```python
from build123d import *

# Parameters (mm, degrees)
F1_DEPTH = 15
F2_W     = 12
F2_H     = 14
F3_DEPTH = 7.5
F4_W     = 11
F4_H     = 14
F5_DEPTH = 17
F6_W     = 11
F6_H     = 1.5
F7_DEPTH = 5.2


with BuildPart() as f1:
    # F0 (on Right) → F1 (new body)
    with BuildSketch(Plane.YZ):
        Polygon((-17, 0), (0, 0), (0, 7.5), (-4, 7.5), (-4, 17), (-8.5, 17), (-8.5, 14), (-6, 14), (-6, 10), (-11.8, 10), (-11.8, 17), (-17, 11.8), align=None)
    extrude(amount=F1_DEPTH)

    # F2 (on face) → F3 (cut)
    with BuildSketch(Plane(origin=(0, 0, 0), x_dir=(1, 0, 0), z_dir=(0, 0, -1))):
        with Locations((7.5, 8.5)):
            Rectangle(F2_W, F2_H)
    extrude(amount=-F3_DEPTH, mode=Mode.SUBTRACT)

    # F4 (on face) → F5 (cut)
    with BuildSketch(Plane.XY.offset(17)):
        with Locations((7.5, -8.5)):
            Rectangle(F4_W, F4_H)
    extrude(amount=-F5_DEPTH, mode=Mode.SUBTRACT)

    # F6 (on face) → F7 (cut)
    with BuildSketch(Plane.XY.offset(17)):
        with Locations((7.5, -16.25)):
            Rectangle(F6_W, F6_H)
    extrude(amount=-F7_DEPTH, mode=Mode.SUBTRACT)


solid = f1.part
```
Source: CAD feature listing. Evaluate the final solid. Frame: model axes, mm. A direction names the side the tool comes from. Coordinates: 2 decimals unless noted, no trailing zeros. Order: outer loops, then holes, each group sorted by start corner. A loop starts at its lowest first (then second) coordinate and runs counter-clockwise, first axis right, second up. Notation, with made-up numbers: M 36.25,70 L 71.25,70 A15 ccw 71.25,78 Z; hole C 18,75.5 d11. An arc over 180 degrees is marked long. Write each question's results on one line, items separated by ' | '. Start each with the question number.
1) Section query B-B (x = 2.25). Return the cut outline in (y, z), plus the area to 4 significant figures.
2) Draft query along X for faces 1 (the face through (0, -9, 7)), 2 (the face through (2, -12, 11)), 3 (the face through (1, -11.8, 13)). Return one class per face: released by +X, released by -X, zero draft, split by the parting line, or undercut.
3) Access query for faces 4 (the face through (14, -4, 12)), 5 (the face through (13.5, -8, 4)), 6 (the face through (14, -7, 14)), 7 (the face through (14, -11.8, 13)). Directions: +Z, -Z, +X, -X, +Y, -Y. A direction counts if a zero-diameter tool reaches every point of the face in a straight line with its end or side. Return the directions, or none.
4) Contact query for flat-ended pins moving along their axis: pin 1 Ø1 at (x, y) = (0.5, -10) entering from +Z; pin 2 Ø1.2 at (x, y) = (5, -1.5) entering from +Z; pin 3 Ø0.6 at (x, z) = (14.5, 15.5) entering from -Y. Output: stop coordinate, or through.
5) Section query D-D (z = 1.5). Return the cut outline in (x, y), plus the area to 3 significant figures.
6) Section query C-C (z = 12.5). Return the cut outline in (x, y).
7) Line query: line 1 (X direction, y = -9.5, z = 3); line 2 (X direction, y = -4.25, z = 15); line 3 (Y direction, x = 5.75, z = 3.25). Output: solid intervals per line, ascending. Write a range as from..to.
8) Section query A-A (y = -2). Return the cut outline in (x, z).
Answers:
1) outline: M -17,0 L -15.5,0 L -15.5,11.8 L -17,11.8 Z; M -1.5,0 L 0,0 L 0,7.5 L -1.5,7.5 Z | area: 28.95 mm^2
2) face 1: released by -X | face 2: undercut | face 3: zero draft
3) face 4: +Z, +X, -X, +Y | face 5: -Z | face 6: +X, -X | face 7: +Z, +X, -X
4) pin 1: stops at z = 10 | pin 2: stops at z = 7.5 | pin 3: stops at y = -13.6
5) outline: M 0,-17 L 15,-17 L 15,0 L 0,0 Z; hole M 1.5,-15.5 L 13.5,-15.5 L 13.5,-1.5 L 1.5,-1.5 Z | area: 87.0 mm^2
6) outline: M 0,-16.3 L 2,-16.3 L 2,-11.8 L 0,-11.8 Z; M 0,-6 L 2,-6 L 2,-4 L 0,-4 Z; M 13,-16.3 L 15,-16.3 L 15,-11.8 L 13,-11.8 Z; M 13,-6 L 15,-6 L 15,-4 L 13,-4 Z
7) line 1: x = 0..1.5, 13.5..15 | line 2: x = 0..2, 13..15 | line 3: y = -17..-15.5, -1.5..0
8) outline: M 0,0 L 1.5,0 L 1.5,7.5 L 0,7.5 Z; M 13.5,0 L 15,0 L 15,7.5 L 13.5,7.5 Z
